Verification items for the finished model (mm, model axes). A direction names the side the tool comes from. Coordinates: 2 decimals unless noted, no trailing zeros. Write each loop counter-clockwise with the first axis right and the second up, starting at its lowest first coordinate (ties: lowest second). Pieces come first, ordered by that corner, then holes. Notation, with made-up numbers: (14, 51) - (59, 51) arc R22 cw to (59, 72) - close; hole circle Ø4 at (50.25, -2.5). An arc over 180 degrees is marked (long way). Use one line per item in the form item = value. Start each with the question number.
(1) Sectioned sample at C-C (y = 46.5). Record the cut outline in (x, z), and give its area (3 significant figures).
(2) Tool access check on faces 1 (the flat face through (1, 61, 25)), 2 (the flat face through (13, 49, 90)), 3 (the flat face through (15, 21, 56)), 4 (the flat face through (-41, 30, 77)). Record the directions out of +Z, -Z, +X, -X, +Y, -Y that give a thin tool (end or side, any length) a straight path to the whole face; none if there is none.
(3) Gauge pin test, flat ends, axial feed: pin 1 Ø3 at (x, z) = (2.5, 90.5) entering from +Y; pin 2 Ø6 at (x, z) = (14, 63.5) entering from -Y; pin 3 Ø23 at (x, y) = (-9.5, 7) entering from +Z; pin 4 Ø1.8 at (x, y) = (-50, 8.5) entering from -Z. Record the tip position at first contact, or that the pin passes through.
(4) Sectioned sample at B-B (x = 50). Record the cut outline in (y, z), and give its area (3 significant figures).
(5) Sectioned sample at D-D (y = 26.5). Record the cut outline in (x, z).
(6) Mould release check, pull along Z, two halves, no side actions. Record for faces 5 (the flat face through (1, 72, 10)), 6 (the flat face through (13, 51, 95)), 7 (the flat face through (13, 54, 97)), 8 (the flat face through (13, 36, 62)): released by +Z, released by -Z, zero draft, split by the parting line, or undercut.
(7) Material ranges on line 1 (X direction, y = 73.5, z = 6.75); line 2 (Y direction, x = -50, z = 4.75); line 3 (Z direction, x = 50.5, y = 42.5), recorded low to high. Write a range as [from, to].
(8) Sectioned sample at A-A (y = 73.5). Record the cut outline in (x, z), and give its area (3 significant figures).
from build123d import *

# Parameters (mm, degrees)
F1_DEPTH      = 65
F1_DEPTH_BACK = 65
F3_DEPTH      = 106
F4_R          = 1.5
F5_DEPTH      = 10


with BuildPart() as f1:
    # F0 (on Right) → F1 (new body, two sides)
    with BuildSketch(Plane.YZ) as f1_sk:
        Polygon((0, 10), (0, 0), (82, 0), (82, 10), (61, 10), (61, 40), (21, 40), (21, 10), align=None)
    extrude(amount=F1_DEPTH)
    extrude(f1_sk.sketch, amount=-F1_DEPTH_BACK)

    # F2 (on face) → F3 (join)
    with BuildSketch(Plane.YZ.offset(65)):
        Polygon((21, 100), (21, 40), (36, 40), (36, 85), (49, 85), (49, 95), (54, 95), (54, 100), align=None)
    extrude(amount=-F3_DEPTH)

    # F4 (on face) → F5 (cut)
    with BuildSketch(Plane.XY.offset(10)):
        with Locations((-50, 73.5)):
            Circle(F4_R)
        with Locations((0, 73.5)):
            Circle(F4_R)
        with Locations((50, 73.5)):
            Circle(F4_R)
        with Locations((50, 8.5)):
            Circle(F4_R)
        with Locations((0, 8.5)):
            Circle(F4_R)
        with Locations((-50, 8.5)):
            Circle(F4_R)
    extrude(amount=-F5_DEPTH, mode=Mode.SUBTRACT)


solid = f1.part
Answers below:
q1.outline = (-65, 0) - (65, 0) - (65, 40) - (-65, 40) - close; (-41, 85) - (65, 85) - (65, 100) - (-41, 100) - close
q1.area = 6,790 mm2
q2.face_1 = +Z, +X, -X, +Y
q2.face_2 = +X, -X, +Y
q2.face_3 = +Z, +X, -X, -Y
q2.face_4 = +Z, -X, +Y, -Y
q3.pin_1 = 49
q3.pin_2 = 21
q3.pin_3 = 10
q3.pin_4 = through
q4.outline = (0, 0) - (7, 0) - (7, 10) - (0, 10) - close; (10, 0) - (72, 0) - (72, 10) - (61, 10) - (61, 40) - (36, 40) - (36, 85) - (49, 85) - (49, 95) - (54, 95) - (54, 100) - (21, 100) - (21, 10) - (10, 10) - close; (75, 0) - (82, 0) - (82, 10) - (75, 10) - close
q4.area = 3,080 mm2
q5.outline = (-65, 0) - (65, 0) - (65, 100) - (-41, 100) - (-41, 40) - (-65, 40) - close
q6.face_5 = released by +Z
q6.face_6 = undercut
q6.face_7 = zero draft
q6.face_8 = undercut
q7.line_1 = [-65, -51.5], [-48.5, -1.5], [1.5, 48.5], [51.5, 65]
q7.line_2 = [0, 7], [10, 72], [75, 82]
q7.line_3 = [0, 40], [85, 100]
q8.outline = (-65, 0) - (-51.5, 0) - (-51.5, 10) - (-65, 10) - close; (-48.5, 0) - (-1.5, 0) - (-1.5, 10) - (-48.5, 10) - close; (1.5, 0) - (48.5, 0) - (48.5, 10) - (1.5, 10) - close; (51.5, 0) - (65, 0) - (65, 10) - (51.5, 10) - close
q8.area = 1,210 mm2
